from build123d import *

# Parameters (mm, degrees)
SKETCH_1_R          = 2.2
EXTRUDE_1_DEPTH     = 4
SKETCH_2_R          = 1.5
EXTRUDE_2_DEPTH     = 2
FILLET_1_R          = 3
SKETCH_3_W          = 10
SKETCH_3_H          = 1
CUT_EXTRUDE_1_DEPTH = 10


with BuildPart() as part:
    # 草图1 → 凸台-拉伸1 (new body)
    with BuildSketch(Plane.XY):
        Polygon((-4.975166703, 0), (-4.975166703, -8), (5.024833297, -8), (5.024833297, 0), (5.024833297, 5), (-4.975166703, 5), align=None)
        Circle(SKETCH_1_R, mode=Mode.SUBTRACT)
    extrude(amount=EXTRUDE_1_DEPTH)

    # 草图2 → 凸台-拉伸2 (add)
    with BuildSketch(Plane.XZ.offset(8)):
        Polygon((5.024833297, 0), (5.024833297, -18), (-4.975166703, -18), (-4.975166703, 21), (5.024833297, 21), align=None)
        with Locations(Location((0, -13, 0), (0, 0, 270))):
            Circle(SKETCH_2_R, mode=Mode.SUBTRACT)
        with Locations(Location((0, 16, 0), (0, 0, 90))):
            Circle(SKETCH_2_R, mode=Mode.SUBTRACT)
    extrude(amount=EXTRUDE_2_DEPTH)

    # 圆角1
    fillet_1_edges = [part.edges().sort_by_distance(p)[0] for p in [
        (-4.975166703, 5, 2),
        (5.024833297, 5, 2),
    ]]
    fillet(fillet_1_edges, radius=FILLET_1_R)

    # 草图3 → 切除-拉伸1 (cut)
    with BuildSketch(Plane.XZ.offset(10)):
        with Locations((0.024833297, 20.5)):
            Rectangle(SKETCH_3_W, SKETCH_3_H)
        with Locations((0.024833297, -17.5)):
            Rectangle(SKETCH_3_W, SKETCH_3_H)
    extrude(amount=-CUT_EXTRUDE_1_DEPTH, mode=Mode.SUBTRACT)


solid = part.part
CAD build for the part. Positions are in the model's coordinates, mm. A direction names the side the tool comes from. Coordinates: 2 decimals unless noted, no trailing zeros. Order: outer loops, then holes, each group sorted by start corner. A loop starts at its lowest first (then second) coordinate and runs counter-clockwise, first axis right, second up. Notation, with made-up numbers: (-23, -14.75) -> (9, -14.75) arc R23 ccw to (9, -5.75) -> close; hole circle Ø1 at (42, 41). An arc over 180 degrees is marked (long way). Answer in a Markdown table with one row per item.
1) Band-saw the part on D-D (z = 0.5). List the corners of the cut face in (x, y).
Check values:
| item | result |
|---|---|
| outline | (-4.98, -10) -> (5.02, -10) -> (5.02, 2) arc R3 ccw to (2.02, 5) -> (-1.98, 5) arc R3 ccw to (-4.98, 2) -> close; hole circle Ø4.4 at (0, 0) |
2) Which spindle directions (+Z, -Z, +X, -X, +Y, -Y) get a long thin tool onto all of the face, cutting with end or side? Do faces 4 (the face through (0, -8, -8)), 5 (the face through (0, -8, 12)), 6 (the face through (0, -10, 2)). Say none if no direction does.
Check values:
| item | result |
|---|---|
| face 4 | -Z, +X, -X, +Y |
| face 5 | +Z, +X, -X, +Y |
| face 6 | +Z, -Z, +X, -X, -Y |
3) Band-saw the part on A-A (z = 16). List the corners of the cut face in (x, y), and give its area (3 significant figures).
Check values:
| item | result |
|---|---|
| outline | (-4.98, -10) -> (-1.5, -10) -> (-1.5, -8) -> (-4.98, -8) -> close; (1.5, -10) -> (5.02, -10) -> (5.02, -8) -> (1.5, -8) -> close |
| area | 14.0 mm2 |
4) Mould opens along Z. For faces 1 (the face through (0, -3, 4)), 2 (the face through (4.17, 4.1, 2.03)), 3 (the face through (0.07, -8.99, -11.5)) say: pulls with the +Z half, pulls with the -Z half, needs draft (parallel to the pull), parting line crosses it, or undercut.
Check values:
| item | result |
|---|---|
| face 1 | pulls with the +Z half |
| face 2 | needs draft |
| face 3 | undercut |
5) Band-saw the part on C-C (x = 0). List the corners of the cut face in (y, z).
Check values:
| item | result |
|---|---|
| outline | (-10, -17) -> (-8, -17) -> (-8, -14.5) -> (-10, -14.5) -> close; (-10, -11.5) -> (-8, -11.5) -> (-8, 0) -> (-2.2, 0) -> (-2.2, 4) -> (-8, 4) -> (-8, 14.5) -> (-10, 14.5) -> close; (-10, 17.5) -> (-8, 17.5) -> (-8, 20) -> (-10, 20) -> close; (2.2, 0) -> (5, 0) -> (5, 4) -> (2.2, 4) -> close |
6) Drill centre lines: line 1 (X direction, y = -8.65, z = -13); line 2 (Y direction, x = 1, z = -11); line 3 (Z direction, x = 4, y = 3). Where is each one in solid material? Low to high.
Check values:
| item | result |
|---|---|
| line 1 | -4.98 to -1.5, 1.5 to 5.02 |
| line 2 | -10 to -8 |
| line 3 | 0 to 4 |
7) Band-saw the part on B-B (y = 0). List the corners of the cut face in (x, z), and give its area (3 significant figures).
Check values:
| item | result |
|---|---|
| outline | (-4.98, 0) -> (-2.2, 0) -> (-2.2, 4) -> (-4.98, 4) -> close; (2.2, 0) -> (5.02, 0) -> (5.02, 4) -> (2.2, 4) -> close |
| area | 22.4 mm2 |
8) Flat gauge pins, fed straight in: P1, Ø1, axis at x = 2.5, y = 1, coming from the -Z side; P2, Ø4, axis at x = 2, y = -5, coming from the +Z side; P3, Ø1, axis at x = -4, z = -12, coming from the +Y side. Where does each tip first touch, or does it go through?
Check values:
| item | result |
|---|---|
| P1 | z = 0 |
| P2 | z = 4 |
| P3 | y = -8 |
